Autodesk Fusion 360 part; units mm, degrees
sketch "Skizze1" plane through (0, 0, 0) normal (0, 0, 1) x (1, 0, 0)
  line L0 (19.25, -19.75) -> (-19.25, -19.75)
  line L1 (-19.25, -19.75) -> (-19.25, 19.75)
  line L2 (-19.25, 19.75) -> (19.25, 19.75)
  line L3 (19.25, 19.75) -> (19.25, -19.75)
  line L4 (19.25, -19.75) -> (-19.25, 19.75) construction
  line L5 (-19.25, -19.75) -> (19.25, 19.75) construction
  dimension "d1" = 38.5
  dimension "d2" = 39.5
extrude "Extrusion1" add sketch "Skizze1" along normal blind 7.5
sketch "Skizze2" plane through (0, 0, 7.5) normal (0, 0, 1) x (-1, 0, 0)
  line L0 (-19.25, -19.75) -> (19.25, -19.75)
  line L1 (19.25, -19.75) -> (19.25, 19.75)
  line L2 (19.25, 19.75) -> (-19.25, 19.75)
  line L3 (-19.25, 19.75) -> (-19.25, -19.75)
  line L4 (16.75, 17.25) -> (-17.75, 17.25)
  line L5 (-17.75, 17.25) -> (-17.75, -17.25)
  line L6 (-17.75, -17.25) -> (16.75, -17.25)
  line L7 (16.75, -17.25) -> (16.75, 17.25)
  dimension "d5" = 2.5
  dimension "d6" = 2.5
  dimension "d7" = 2.5
extrude "Extrusion2" cut sketch "Skizze2" against normal blind 1 contours L4 L5 L6 L7
sketch "Skizze3" plane through (0, 0, 0) normal (0, 0, -1) x (1, 0, 0)
  line L0 (-19.25, -19.75) -> (19.25, -19.75)
  line L1 (19.25, -19.75) -> (19.25, 19.75)
  line L2 (19.25, 19.75) -> (-19.25, 19.75)
  line L3 (-19.25, 19.75) -> (-19.25, -19.75)
  line L4 (-16.75, -17.25) -> (17.75, -17.25)
  line L5 (-16.75, 17.25) -> (-16.75, -17.25)
  line L6 (17.75, 17.25) -> (-16.75, 17.25)
  line L7 (17.75, -17.25) -> (17.75, 17.25)
extrude "Extrusion3" cut sketch "Skizze3" against normal blind 0.6 contours L4 L5 L6 L7
sketch "Skizze4" plane through (0, 0, 6.5) normal (0, 0, 1) x (-1, 0, 0)
  line L0 (16.75, -17.25) -> (16.75, 17.25)
  line L1 (16.75, 17.25) -> (-17.75, 17.25)
  line L2 (-17.75, 17.25) -> (-17.75, -17.25)
  line L3 (-17.75, -17.25) -> (16.75, -17.25)
  line L4 (15.25, -15.75) -> (-16.25, -15.75)
  line L5 (-16.25, -15.75) -> (-16.25, 15.75)
  line L6 (-16.25, 15.75) -> (15.25, 15.75)
  line L7 (15.25, 15.75) -> (15.25, -15.75)
  line L8 (14.105, -14.605) -> (-15.105, -14.605) construction
  line L9 (-15.105, -14.605) -> (-15.105, 14.605) construction
  line L10 (-15.105, 14.605) -> (14.105, 14.605) construction
  line L11 (14.105, 14.605) -> (14.105, -14.605) construction
  line L12 (14.105, -14.605) -> (16.75, -17.25) construction
  line L13 (14.105, 14.605) -> (16.75, 17.25) construction
  line L14 (14.105, -11.605) -> (15.25, -11.605)
  line L15 (11.105, -14.605) -> (11.105, -15.75)
  line L16 (-12.105, -14.605) -> (-12.105, -15.75)
  line L17 (-15.105, -11.605) -> (-16.25, -11.605)
  line L18 (-15.105, 11.605) -> (-16.25, 11.605)
  line L19 (-12.105, 14.605) -> (-12.105, 15.75)
  line L20 (14.105, 11.605) -> (15.25, 11.605)
  line L21 (11.105, 14.605) -> (11.105, 15.75)
  arc A0 (11.105, 14.605) -> (14.105, 11.605) centre (14.105, 14.605) ccw
  arc A1 (14.105, -11.605) -> (11.105, -14.605) centre (14.105, -14.605) ccw
  arc A2 (-12.105, -14.605) -> (-15.105, -11.605) centre (-15.105, -14.605) ccw
  arc A3 (-15.105, 11.605) -> (-12.105, 14.605) centre (-15.105, 14.605) ccw
  dimension "d12" = 1.5
  dimension "d13" = 1.5
  dimension "d14" = 1.5
  dimension "d15" = 1.5
  dimension "d16" = 6
  dimension "d17" = 29.21
extrude "Extrusion4" cut sketch "Skizze4" against normal through all contours L4 L5 L6 L7 L14 L15 L16 L17 L18 L19 L20 L21 A0 A1 A2 A3
sketch "Skizze5" plane through (0, 0, 6.5) normal (0, 0, 1) x (-1, 0, 0)
  line L0 (-12.105, 15.75) -> (11.105, 15.75)
  line L1 (11.105, 15.75) -> (11.105, 14.605)
  arc A0 (11.105, 14.605) -> (14.105, 11.605) centre (14.105, 14.605) ccw
  line L2 (14.105, 11.605) -> (15.25, 11.605)
  line L3 (15.25, 11.605) -> (15.25, -11.605)
  line L4 (15.25, -11.605) -> (14.105, -11.605)
  arc A1 (14.105, -11.605) -> (11.105, -14.605) centre (14.105, -14.605) ccw
  line L5 (11.105, -14.605) -> (11.105, -15.75)
  line L6 (11.105, -15.75) -> (-12.105, -15.75)
  line L7 (-12.105, -15.75) -> (-12.105, -14.605)
  arc A2 (-12.105, -14.605) -> (-15.105, -11.605) centre (-15.105, -14.605) ccw
  line L8 (-15.105, -11.605) -> (-16.25, -11.605)
  line L9 (-16.25, -11.605) -> (-16.25, 11.605)
  line L10 (-16.25, 11.605) -> (-15.105, 11.605)
  arc A3 (-15.105, 11.605) -> (-12.105, 14.605) centre (-15.105, 14.605) ccw
  line L11 (-12.105, 14.605) -> (-12.105, 15.75)
  line L12 (16.75, -17.25) -> (16.75, 17.25)
  line L13 (16.75, 17.25) -> (-17.75, 17.25)
  line L14 (-17.75, 17.25) -> (-17.75, -17.25)
  line L15 (-17.75, -17.25) -> (16.75, -17.25)
  circle A4 centre (14.105, -14.605) radius 1.25
  circle A5 centre (14.105, 14.605) radius 1.25
  circle A6 centre (-15.105, -14.605) radius 1.25
  circle A7 centre (-15.105, 14.605) radius 1.25
  dimension "d19" = 2.5
extrude "Extrusion5" cut sketch "Skizze5" against normal through all contours A4 | A5 | A6 | A7
sketch "Skizze6" plane through (0, 0, 7.5) normal (0, 0, 1) x (-1, 0, 0)
  line L0 (-17.75, 17.25) -> (16.75, 17.25)
  line L1 (16.75, 17.25) -> (16.75, -17.25)
  line L2 (16.75, -17.25) -> (-17.75, -17.25)
  line L3 (-17.75, -17.25) -> (-17.75, 17.25)
  line L4 (-19.25, -19.75) -> (19.25, -19.75)
  line L5 (19.25, -19.75) -> (19.25, 19.75)
  line L6 (19.25, 19.75) -> (-19.25, 19.75)
  line L7 (-19.25, 19.75) -> (-19.25, -19.75)
  line L8 (16.75, -11.25) -> (19.25, -11.25)
  line L9 (19.25, -11.25) -> (19.25, -3.75)
  line L10 (19.25, -3.75) -> (16.75, -3.75)
  line L11 (16.75, -3.75) -> (16.75, -11.25)
  line L12 (16.75, 3.75) -> (19.25, 3.75)
  line L13 (19.25, 3.75) -> (19.25, 11.25)
  line L14 (19.25, 11.25) -> (16.75, 11.25)
  line L15 (16.75, 11.25) -> (16.75, 3.75)
  line L16 (19.25, -3.75) -> (19.25, 3.75) construction
  dimension "d21" = 7.5
  dimension "d22" = 15
extrude "Extrusion6" add sketch "Skizze6" along normal blind 1 contours L1 L5 L12 L13 L14 L15 | L1 L5 L8 L9 L10 L11
sketch "Skizze7" plane through (0, 0, 0) normal (0, 0, -1) x (1, 0, 0)
  line L0 (-16.75, 17.25) -> (17.75, 17.25)
  line L1 (17.75, 17.25) -> (17.75, -17.25)
  line L2 (17.75, -17.25) -> (-16.75, -17.25)
  line L3 (-16.75, -17.25) -> (-16.75, 17.25)
  line L4 (-19.25, -19.75) -> (19.25, -19.75)
  line L5 (19.25, -19.75) -> (19.25, 19.75)
  line L6 (19.25, 19.75) -> (-19.25, 19.75)
  line L7 (-19.25, 19.75) -> (-19.25, -19.75)
  line L8 (17.75, 17.25) -> (19.25, 17.25)
  line L9 (19.25, 17.25) -> (19.25, -17.25)
  line L10 (19.25, -17.25) -> (17.75, -17.25)
  line L11 (17.75, -17.25) -> (17.75, 17.25)
extrude "Extrusion7" cut sketch "Skizze7" against normal up to surface (0.6 mm away) contours L1 L5 L8 L9 L10 L11
equation "d7 = d6"
equation "d13 = d12"
equation "d14 = d12"
equation "d15 = d12"
Here's how the part is built. I have some questions about the finished solid (model axes, mm). A direction names the side the tool comes from. Give positions to 0.01 mm unless a question says otherwise; leave off trailing zeros. Loops run counter-clockwise (first coordinate to the right, second up) from the corner with the lowest first, then second, coordinate; pieces in that order, holes last. Notation, with made-up numbers: (51.5, 7) -> (92.5, 7) arc R6 ccw to (92.5, 17) -> close; hole circle Ø1 at (45.25, 24.5). An arc over 180 degrees is marked (long way). Use one line per item in the form item = value. Start each with the question number.
1) Please list where these lines run through material, in increasing order: line 1 along Y through (x, z) = (15, 2.75); line 2 along Y through (x, z) = (1, 1.25); line 3 along X through (y, z) = (8, 3.25).
2) Which directions (+Z, -Z, +X, -X, +Y, -Y) give clear straight access to the entire face, cutting with the end or side of a thin tool? Please do faces 1 (the face through (1, 17.25, 7)), 2 (the face through (12.105, 15, 4)), 3 (the face through (-18, 7, 8.5)), 4 (the face through (-18, 0, 7.5)).
3) Imagine slicing it at B-B (x = -4). Please give me the cut outline in (y, z).
4) Imagine slicing it at A-A (y = -4.5). Please give me the cut outline in (x, z).
5) Imagine slicing it at D-D (z = 2). Please give me the cut outline in (x, y) (3 decimals), then the cut area to 3 significant figures.
6) Thinking about a two-plate mould opening in X: for faces 5 (the face through (0, 18, 7.5)), 6 (the face through (-19.25, 0, 4)), 7 (the face through (-15, 11.605, 4)), which applies, +X half, -X half, draft (parallel to the pull), parting line (faces both ways), or undercut?
7) For P1, Ø3, axis at x = 15.105, y = 14.605, coming from the -Z side; P2, Ø0.5, axis at x = -18.5, z = 8, coming from the -Y side; P3, Ø6, axis at x = -9, y = 12.5, coming from the +Z side, each with a flat end and sliding along its axis, tell me the tip position at first contact or that it passes through.
8) Imagine slicing it at C-C (z = 7). Please give me the cut outline in (x, y), then the cut area to 4 significant figures.
Check values:
q1.line_1 = -19.75 to -15.85, -13.36 to -11.61, 11.61 to 13.36, 15.85 to 19.75
q1.line_2 = -19.75 to -15.75, 15.75 to 19.75
q1.line_3 = -19.25 to -15.25, 16.25 to 19.25
q2.face_1 = +Z
q2.face_2 = +Z, -Z
q2.face_3 = +Z, +X, -X, +Y, -Y
q2.face_4 = +Z, +X, -X
q3.outline = (-19.75, 0) -> (-17.25, 0) -> (-17.25, 0.6) -> (-15.75, 0.6) -> (-15.75, 6.5) -> (-17.25, 6.5) -> (-17.25, 7.5) -> (-19.75, 7.5) -> close; (15.75, 0.6) -> (17.25, 0.6) -> (17.25, 0) -> (19.75, 0) -> (19.75, 7.5) -> (17.25, 7.5) -> (17.25, 6.5) -> (15.75, 6.5) -> close
q4.outline = (-19.25, 0) -> (-16.75, 0) -> (-16.75, 0.6) -> (-15.25, 0.6) -> (-15.25, 6.5) -> (-16.75, 6.5) -> (-16.75, 8.5) -> (-19.25, 8.5) -> close; (16.25, 0.6) -> (19.25, 0.6) -> (19.25, 7.5) -> (17.75, 7.5) -> (17.75, 6.5) -> (16.25, 6.5) -> close
q5.outline = (-19.25, -19.75) -> (19.25, -19.75) -> (19.25, 19.75) -> (-19.25, 19.75) -> close; hole circle Ø2.5 at (-14.105, -14.605); hole circle Ø2.5 at (-14.105, 14.605); hole (-15.25, -11.605) -> (-14.105, -11.605) arc R3 cw to (-11.105, -14.605) -> (-11.105, -15.75) -> (12.105, -15.75) -> (12.105, -14.605) arc R3 cw to (15.105, -11.605) -> (16.25, -11.605) -> (16.25, 11.605) -> (15.105, 11.605) arc R3 cw to (12.105, 14.605) -> (12.105, 15.75) -> (-11.105, 15.75) -> (-11.105, 14.605) arc R3 cw to (-14.105, 11.605) -> (-15.25, 11.605) -> close; hole circle Ø2.5 at (15.105, -14.605); hole circle Ø2.5 at (15.105, 14.605)
q5.area = 570 mm^2
q6.face_5 = draft
q6.face_6 = -X half
q6.face_7 = undercut
q7.P1 = 0.6
q7.P2 = -11.25
q7.P3 = 6.5
q8.outline = (-19.25, -19.75) -> (19.25, -19.75) -> (19.25, 19.75) -> (-19.25, 19.75) -> close; hole (-16.75, -17.25) -> (17.75, -17.25) -> (17.75, 17.25) -> (-16.75, 17.25) -> close
q8.area = 330.5 mm^2
